Model file for the job. Use its own axes, mm. A direction names the side the tool comes from. Round coordinates to 2 decimals unless told otherwise and drop trailing zeros. Loops run counter-clockwise (first coordinate to the right, second up) from the corner with the lowest first, then second, coordinate; pieces in that order, holes last. Notation, with made-up numbers: (88.25, 39) - (133.25, 39) arc R27 ccw to (133.25, 72) - close; hole circle Ø2 at (16, 24). An arc over 180 degrees is marked (long way). Answer as a JSON object with one key per item and string values.
from build123d import *

# Parameters (mm, degrees)
ESBO_O1_W                = 174.2
ESBO_O1_H                = 90
RESSALTO_EXTRUS_O1_DEPTH = 10
ESBO_O2_W                = 194.2
ESBO_O2_H                = 110
ESBO_O2_W_2              = 184.2
ESBO_O2_H_2              = 100
RESSALTO_EXTRUS_O2_DEPTH = 20
ESBO_O3_W                = 194.2
ESBO_O3_H                = 110
RESSALTO_EXTRUS_O3_DEPTH = 5
ESBO_O5_R                = 3
CORTE_EXTRUS_O1_DEPTH    = 20
ESBO_O6_W                = 63.181422492
ESBO_O6_H                = 3
RESSALTO_EXTRUS_O4_DEPTH = 17
ESBO_O7_W                = 70
ESBO_O7_H                = 2
ESBO_O7_W_2              = 58
ESBO_O7_H_2              = 3
RESSALTO_EXTRUS_O5_DEPTH = 10
ESBO_O10_W               = 37.92
ESBO_O10_H               = 15
CORTE_EXTRUS_O2_DEPTH    = 75
CORTE_EXTRUS_O3_DEPTH    = 20
ESBO_O13_W               = 184.2
ESBO_O13_H               = 100
ESBO_O13_W_2             = 174.2
ESBO_O13_H_2             = 90
RESSALTO_EXTRUS_O6_DEPTH = 10
RESSALTO_EXTRUS_O7_DEPTH = 10
ESBO_O17_W               = 194.2
ESBO_O17_H               = 10
CORTE_EXTRUS_O5_DEPTH    = 200


with BuildPart() as part:
    # Esbo_o1 → Ressalto-extrus_o1 (new body)
    with BuildSketch(Plane.XY):
        with Locations((14.940102366, -12.259532062)):
            Rectangle(ESBO_O1_W, ESBO_O1_H)
    extrude(amount=RESSALTO_EXTRUS_O1_DEPTH)



with BuildPart() as body_2:
    # Esbo_o2 → Ressalto-extrus_o2 (new body)
    with BuildSketch(Plane(origin=(0, 0, 0), x_dir=(-1, 0, 0), z_dir=(0, 0, -1))):
        with Locations((-14.940102366, -12.259532062)):
            Rectangle(ESBO_O2_W, ESBO_O2_H)
        with Locations((-14.900102366, -12.219532062)):
            Rectangle(ESBO_O2_W_2, ESBO_O2_H_2, mode=Mode.SUBTRACT)
    extrude(amount=-RESSALTO_EXTRUS_O2_DEPTH)


with BuildPart() as part_1:
    add(part.part)

    add(body_2.part)  # Ressalto-extrus_o3 merges body 2
    # Esbo_o3 → Ressalto-extrus_o3 (add)
    with BuildSketch(Plane(origin=(0, 0, 0), x_dir=(-1, 0, 0), z_dir=(0, 0, -1))):
        with Locations((-14.940102366, -12.259532062)):
            Rectangle(ESBO_O3_W, ESBO_O3_H)
    extrude(amount=RESSALTO_EXTRUS_O3_DEPTH)

    # Esbo_o5 → Corte-extrus_o1 (cut)
    with BuildSketch(Plane.XY.offset(10)):
        with Locations((-64.159897634, -12.259532062)):
            Circle(ESBO_O5_R)
        with Locations((94.040102366, -12.259532062)):
            Circle(ESBO_O5_R)
        with Locations((-39.659897634, -12.259532062)):
            Circle(ESBO_O5_R)
        with Locations((69.540102366, -12.259532062)):
            Circle(ESBO_O5_R)
        with Locations((56.540102366, -12.259532062)):
            Circle(ESBO_O5_R)
    extrude(amount=-CORTE_EXTRUS_O1_DEPTH, mode=Mode.SUBTRACT)

    # Esbo_o6 → Ressalto-extrus_o4 (add)
    with BuildSketch(Plane.XY.offset(10)):
        with Locations((-36.569186388, 4.240467938)):
            Rectangle(ESBO_O6_W, ESBO_O6_H)
    extrude(amount=RESSALTO_EXTRUS_O4_DEPTH)

    # Esbo_o7 → Ressalto-extrus_o5 (add)
    with BuildSketch(Plane.XY.offset(10)):
        with Locations((-34.149897634, -41.229786606)):
            Rectangle(ESBO_O7_W, ESBO_O7_H)
        with Locations((-34.149897634, -45.229786606)):
            Rectangle(ESBO_O7_W, ESBO_O7_H)
        with Locations((69.960102366, 17.908396253)):
            Rectangle(ESBO_O7_W_2, ESBO_O7_H_2)
        with Locations((69.960102366, 22.908396253)):
            Rectangle(ESBO_O7_W_2, ESBO_O7_H_2)
    extrude(amount=RESSALTO_EXTRUS_O5_DEPTH)

    # Esbo_o10 → Corte-extrus_o2 (cut)
    with BuildSketch(Plane.XZ.offset(46.229786606)):
        with Locations((73.920102366, 19.5)):
            Rectangle(ESBO_O10_W, ESBO_O10_H)
    extrude(amount=-CORTE_EXTRUS_O2_DEPTH, mode=Mode.SUBTRACT)

    # Esbo_o11 → Corte-extrus_o3 (cut)
    with BuildSketch(Plane.XY.offset(10)):
        with BuildLine():
            Line((81.040102366, -37.559532062), (87.040102366, -37.559532062))
            ThreePointArc((87.040102366, -37.559532062), (91.723412608, -41.863798339), (87.828759302, -46.89289156))
            Line((87.828759302, -46.89289156), (81.040102366, -46.959532062))
            ThreePointArc((81.040102366, -46.959532062), (76.340102366, -42.259532062), (81.040102366, -37.559532062))
        make_face()
    extrude(amount=-CORTE_EXTRUS_O3_DEPTH, mode=Mode.SUBTRACT)

    # Esbo_o13 → Ressalto-extrus_o6 (add)
    with BuildSketch(Plane.XY):
        with Locations((14.900102366, -12.219532062)):
            Rectangle(ESBO_O13_W, ESBO_O13_H)
        with Locations((14.940102366, -12.259532062)):
            Rectangle(ESBO_O13_W_2, ESBO_O13_H_2, mode=Mode.SUBTRACT)
    extrude(amount=RESSALTO_EXTRUS_O6_DEPTH)

    # Esbo_o14 → Ressalto-extrus_o7 (add)
    with BuildSketch(Plane.XY.offset(10)):
        Polygon((101.960102366, -57.179532062), (-72.159897634, -57.179532062), (-72.159897634, -18.299532062), (-68.159897634, -18.299532062), (-68.159897634, -54.179532062), (98.960102366, -54.179532062), (98.960102366, -18.299532062), (101.960102366, -18.299532062), align=None)
        Polygon((101.960102366, 32.740467938), (-72.159897634, 32.740467938), (-72.159897634, -6.219532062), (-68.159897634, -6.219532062), (-68.159897634, 29.740467938), (98.960102366, 29.740467938), (98.960102366, -6.219532062), (101.960102366, -6.219532062), align=None)
    extrude(amount=RESSALTO_EXTRUS_O7_DEPTH)

    # Esbo_o17 → Corte-extrus_o5 (cut)
    with BuildSketch(Plane.XZ.offset(67.259532062)):
        with Locations((14.940102366, 0)):
            Rectangle(ESBO_O17_W, ESBO_O17_H)
    extrude(amount=-CORTE_EXTRUS_O5_DEPTH, mode=Mode.SUBTRACT)


solid = part_1.part
1) Two-plate mould, pull along X, no slides. Class faces 1 (the flat face through (14, -54.18, 15)), 2 (the flat face through (-82.16, -13, 13)), 3 (the flat face through (23, -65, 20)): pulls with the +X half, pulls with the -X half, needs draft (parallel to the pull), parting line crosses it, or undercut.
Values follow:
{"face 1": "undercut", "face 2": "pulls with the -X half", "face 3": "needs draft"}
2) Drop flat-ended pins along their axis: P1, Ø12, axis at x = -20.5, y = -26.5, coming from the +Z side; P2, Ø19.5, axis at x = -21, y = -38, coming from the +Z side; P3, Ø1, axis at x = -26, z = 21.5, coming from the -Y side. Give the stop position or say it passes through.
Values follow:
{"P1": "z = 10", "P2": "z = 20", "P3": "y = 2.74"}
3) Slice it at D-D on x = 22. List the corners of the cut face in (y, z), then the cut area to 3 significant figures.
Values follow:
{"outline": "(-67.26, 5) - (42.74, 5) - (42.74, 20) - (37.78, 20) - (37.78, 10) - (32.74, 10) - (32.74, 20) - (29.74, 20) - (29.74, 10) - (-54.18, 10) - (-54.18, 20) - (-57.18, 20) - (-57.18, 10) - (-62.22, 10) - (-62.22, 20) - (-67.26, 20) - close", "area": "710 mm²"}
4) Probe probe 1 along X at (y, z) = (-30, 17.5); probe 2 along X at (y, z) = (-45, 13.25); probe 3 along Y at (x, z) = (82, 18.25). List the from-to ranges inside material, lowest first.
Values follow:
{"probe 1": "-82.16 to -77.2, -72.16 to -68.16, 98.96 to 101.96, 107 to 112.04", "probe 2": "-82.16 to -77.2, -72.16 to 0.85, 98.96 to 101.96, 107 to 112.04", "probe 3": "-67.26 to -62.22, -57.18 to -54.18, 29.74 to 32.74, 37.78 to 42.74"}
5) Slice it at B-B on z = 17. Count the separate pieces of the cut face and the enclosed holes in it, then the cut area to 3 significant figures.
Values follow:
{"separate pieces": "5", "enclosed holes": "1", "area": "5,080 mm²"}
6) Slice it at A-A on x = -49.5. List the corners of the cut face in (y, z), then the cut area to 3 significant figures.
Values follow:
{"outline": "(-67.26, 5) - (42.74, 5) - (42.74, 20) - (37.78, 20) - (37.78, 10) - (32.74, 10) - (32.74, 20) - (29.74, 20) - (29.74, 10) - (5.74, 10) - (5.74, 27) - (2.74, 27) - (2.74, 10) - (-40.23, 10) - (-40.23, 20) - (-42.23, 20) - (-42.23, 10) - (-44.23, 10) - (-44.23, 20) - (-46.23, 20) - (-46.23, 10) - (-54.18, 10) - (-54.18, 20) - (-57.18, 20) - (-57.18, 10) - (-62.22, 10) - (-62.22, 20) - (-67.26, 20) - close", "area": "801 mm²"}
7) Slice it at C-C on y = -52. List the corners of the cut face in (x, z).
Values follow:
{"outline": "(-82.16, 5) - (112.04, 5) - (112.04, 20) - (107, 20) - (107, 10) - (101.96, 10) - (101.96, 20) - (98.96, 20) - (98.96, 10) - (-68.16, 10) - (-68.16, 20) - (-72.16, 20) - (-72.16, 10) - (-77.2, 10) - (-77.2, 20) - (-82.16, 20) - close"}
8) Tool access for faces 4 (the flat face through (16, 32.74, 15)), 5 (the cylindrical face through (-66.541, -14.085, 7.535)): list every direction of +Z, -Z, +X, -X, +Y, -Y with a clear straight run to the whole face (end or side of a thin tool).
Values follow:
{"face 4": "+Z", "face 5": "+Z, -Z"}
